For this review, take the finished solid that the model builds, in its own axes (mm). Face numbers are marked on the shaded views. A direction names the side the tool comes from. Give positions to 0.01 mm unless a question says otherwise; leave off trailing zeros. Loops run counter-clockwise (first coordinate to the right, second up) from the corner with the lowest first, then second, coordinate; pieces in that order, holes last.
Autodesk Inventor part; units mm, degrees
ref_plane "YZ Plane" through (0, 0, 0) normal (1, 0, 0) x (0, 1, 0)
ref_plane "XZ Plane" through (0, 0, 0) normal (0, 1, 0) x (-1, 0, 0)
ref_plane "XY Plane" through (0, 0, 0) normal (0, 0, 1) x (1, 0, 0)
sketch "Sketch1" plane through (0, 0, 0) normal (0, 0, 1) x (1, 0, 0)
  circle A0 centre (0, 0) radius 2.9629
  point P0 (0, 0)
extrude "Extrusion1" add sketch "Sketch1" against normal blind 50
sketch "Sketch2" plane through (0, 0, 0) normal (0, 0, 1) x (1, 0, 0)
  circle A0 centre (0, 0) radius 2.9629
  point P0 (0, 0)
extrude "Extrusion2" add sketch "Sketch2" along normal blind 50 draft -35
ref_plane "Work Plane1" through (0, 0, 4) normal (0, 0, 1) x (1, 0, 0)
sketch "Sketch3" plane through (0, 0, 4) normal (0, 0, 1) x (1, 0, 0)
  circle A0 centre (0, 0) radius 2.9629
  circle A1 centre (0, 0.134) radius 0.1051
  point P0 (0, 0)
extrude "Extrusion3" add sketch "Sketch3" along normal blind 25 contours A1
sketch "Sketch4" plane through (0, 0.134, 29) normal (0, 0, 1) x (1, 0, 0)
  circle A0 centre (0, 0) radius 0.1051
  point P0 (0, -0.134)
extrude "Extrusion4" add sketch "Sketch4" along normal blind 5 draft 35
sketch "Sketch5" plane through (0, 0.134, 34) normal (0, 0, 1) x (1, 0, 0)
  circle A0 centre (0, 0) radius 3.6062
  point P0 (0, -0.134)
extrude "Extrusion5" add sketch "Sketch5" along normal blind 40
properties part number "00_Laser_coupling"
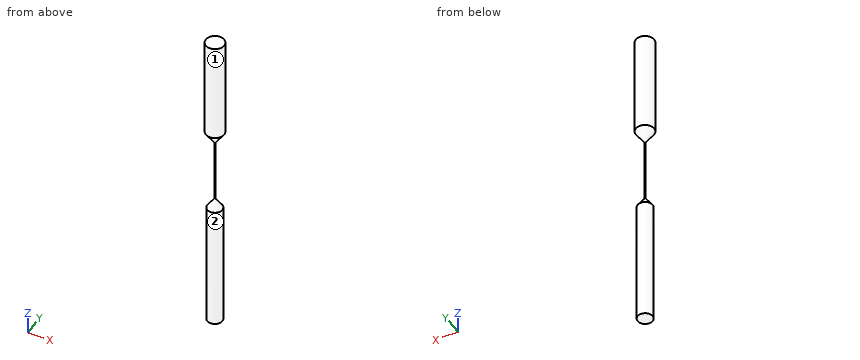
Q1. Consider section A-A on z = 30.5. Give the boundary of the cut face in (x, y).
Answers:
outline: circle Ø2.31 at (0, 0.13)
Q2. For probe 1 along Z at (x, y) = (-2.75, -1); probe 2 along Z at (x, y) = (0.5, -0.5); probe 3 along X at (y, z) = (1, -17.5), list the stretches that pass through material, from the lowest coordinate up.
Answers:
probe 1: z = -50 to 0.05, 33.1 to 74
probe 2: z = -50 to 3.22, 30 to 74
probe 3: x = -2.79 to 2.79
Q3. Machinability: for the marked faces 1 and 2, which of the approach directions +Z, -Z, +X, -X, +Y, -Y give a long, thin tool a straight path to every point of the face, cutting with its end or side? Answer none if there is none.
Answers:
face 1: +Z, -Z
face 2: -Z
